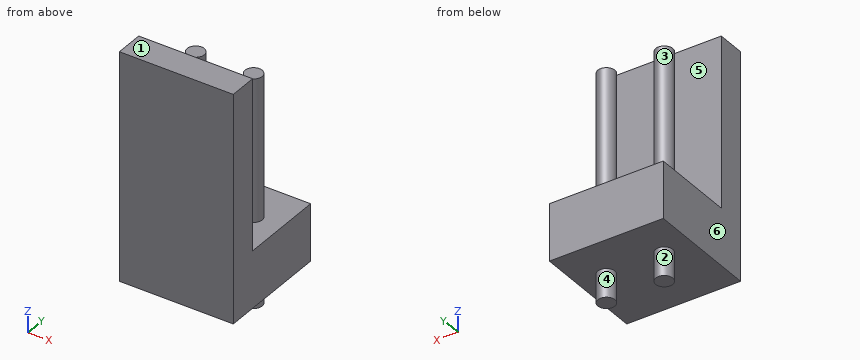
```python
from build123d import *

# Parameters (mm, degrees)
SKETCH_1_W           = 10
SKETCH_1_H           = 10
EXTRUDE_1_DEPTH      = 5
SKETCH_2_W           = 10
SKETCH_2_H           = 2.5
EXTRUDE_2_DEPTH      = 15
EXTRUDE_3_DEPTH      = 12.5
EXTRUDE_3_DEPTH_BACK = 7.5
SKETCH_3_R           = 0.75


with BuildPart() as part:
    # Sketch 1 → Extrude 1 (new body)
    with BuildSketch(Plane.XY):
        with Locations((5, 5)):
            Rectangle(SKETCH_1_W, SKETCH_1_H)
    extrude(amount=EXTRUDE_1_DEPTH)

    # Sketch 2 → Extrude 2 (add)
    with BuildSketch(Plane.XY.offset(5)):
        with Locations((5, 1.25)):
            Rectangle(SKETCH_2_W, SKETCH_2_H)
    extrude(amount=EXTRUDE_2_DEPTH)

    # Sketch 3 → Extrude 3 (add, two sides: drawn at the far end of the back side and taken through both)
    with BuildSketch(Plane.XY.offset(5).offset(-EXTRUDE_3_DEPTH_BACK)):
        with Locations(Location((7.54, 6.25, 0), (0, 0, 180))):
            Circle(SKETCH_3_R)
        with Locations(Location((2.46, 6.25, 0), (0, 0, 180))):
            Circle(SKETCH_3_R)
    extrude(amount=EXTRUDE_3_DEPTH + EXTRUDE_3_DEPTH_BACK)


solid = part.part
```
The listing builds one solid part. Answer for the finished solid, in the listing's coordinates (mm). Face numbers are marked on the shaded views. A direction names the side the tool comes from. Round coordinates to 2 decimals unless told otherwise and drop trailing zeros. Loops run counter-clockwise (first coordinate to the right, second up) from the corner with the lowest first, then second, coordinate; pieces in that order, holes last. Notation, with made-up numbers: (-1.75, 68.5) - (34.25, 68.5) arc R21 ccw to (34.25, 104.5) - close; hole circle Ø11 at (47.25, -40). An arc over 180 degrees is marked (long way). Return JSON: item names as keys, results as strings. Group by question number.
1. The part is cut by section D-D on x = 5. Determine the outline of the cut face in (y, z), then the cut area to 3 significant figures.
2. The part is cut by section B-B on y = 6.25. Determine the outline of the cut face in (x, z).
3. Which of the six approach directions +Z, -Z, +X, -X, +Y, -Y give full straight-line access (tool end or side, diameter ignored) to the marked faces 1, 2 and 3?
4. The part is cut by section A-A on z = 8.75. Determine the outline of the cut face in (x, y).
5. The mould has two halves that part along X. Classify the marked faces 4, 5 and 6: pulls with the +X half, pulls with the -X half, needs draft (parallel to the pull), parting line crosses it, or undercut.
6. Each of these flat-tipped pins is pushed along its axis until it touches: P1, Ø3, axis at x = 4.5, z = 14, coming from the +Y side; P2, Ø4, axis at x = 5, y = 6, coming from the +Z side; P3, Ø1.5, axis at y = 5, z = 7.5, coming from the +X side. Where does it stop, or does it pass through?
7. Consider probe 1 along Y at (x, z) = (3.25, 7.25); probe 2 along Z at (x, y) = (3.25, 7); probe 3 along Z at (x, y) = (7, 6.5). Determine where each line is inside the solid, lowest interval first.
8. The part is cut by section C-C on x = 2.46. Determine the outline of the cut face in (y, z).
Resolved:
{
 "1": {"outline": "(0, 0) - (10, 0) - (10, 5) - (2.5, 5) - (2.5, 20) - (0, 20) - close", "area": "87.5 mm²"},
 "2": {"outline": "(0, 0) - (1.71, 0) - (1.71, -2.5) - (3.21, -2.5) - (3.21, 0) - (6.79, 0) - (6.79, -2.5) - (8.29, -2.5) - (8.29, 0) - (10, 0) - (10, 5) - (8.29, 5) - (8.29, 17.5) - (6.79, 17.5) - (6.79, 5) - (3.21, 5) - (3.21, 17.5) - (1.71, 17.5) - (1.71, 5) - (0, 5) - close"},
 "3": {"face 1": "+Z, +X, -X, +Y, -Y", "face 2": "-Z", "face 3": "+Z"},
 "4": {"outline": "(0, 0) - (10, 0) - (10, 2.5) - (0, 2.5) - close; circle Ø1.5 at (2.46, 6.25); circle Ø1.5 at (7.54, 6.25)"},
 "5": {"face 4": "undercut", "face 5": "needs draft", "face 6": "pulls with the -X half"},
 "6": {"P1": "stops at y = 6.77", "P2": "stops at z = 17.5", "P3": "stops at x = 8.1"},
 "7": {"probe 1": "y = 0 to 2.5", "probe 2": "z = 0 to 5", "probe 3": "z = -2.5 to 17.5"},
 "8": {"outline": "(0, 0) - (5.5, 0) - (5.5, -2.5) - (7, -2.5) - (7, 0) - (10, 0) - (10, 5) - (7, 5) - (7, 17.5) - (5.5, 17.5) - (5.5, 5) - (2.5, 5) - (2.5, 20) - (0, 20) - close"}
}
